The drawing under review shows one solid part. Ordinate dimensions are in mm from its lowest x, y, z. A direction names the side the tool comes from. Give positions to 0.01 mm unless a question says otherwise; leave off trailing zeros. Loops run counter-clockwise (first coordinate to the right, second up) from the corner with the lowest first, then second, coordinate; pieces in that order, holes last.
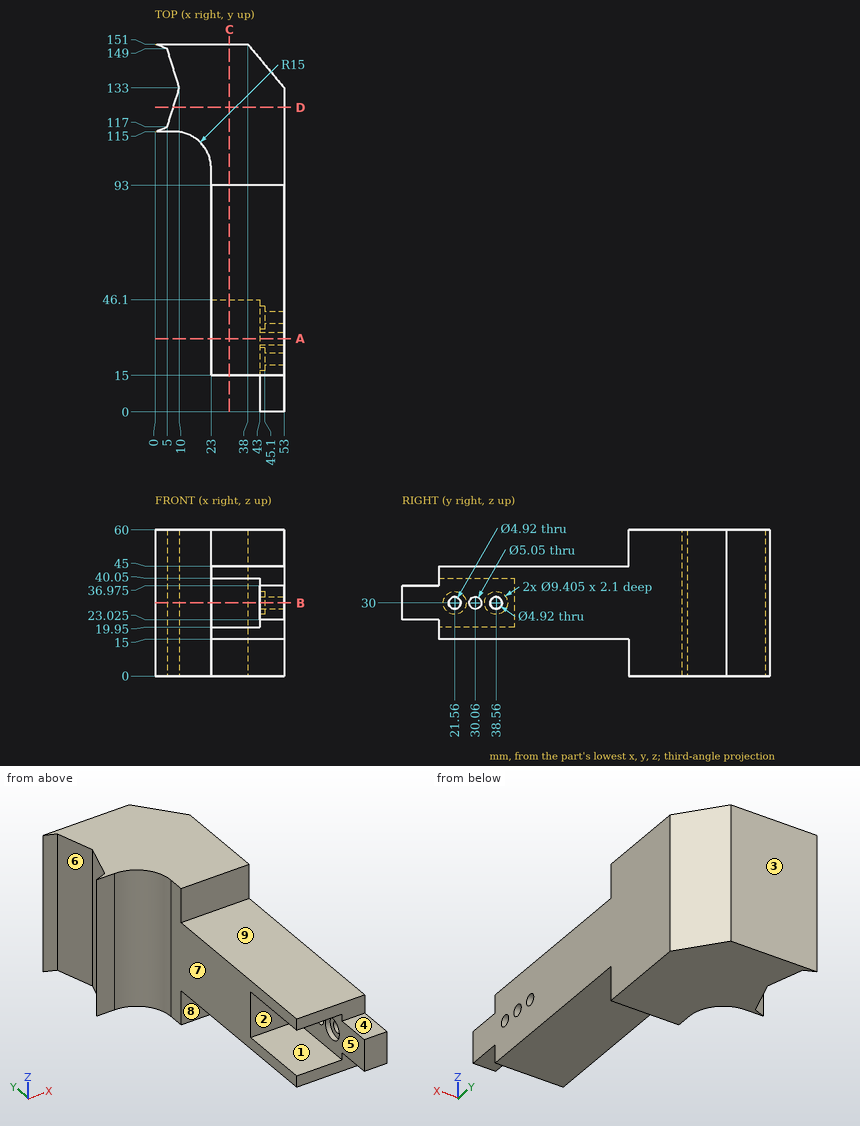
Item 1: Take a section at B-B on z = 30. State how many separate pieces and enclosed holes the cut face has, and give its area (3 significant figures).
Answer:
separate pieces: 4
enclosed holes: 0
area: 3,930 mm2
Item 2: Clearance check with flat-ended pins moving along their axes: pin 1 Ø16 at (x, z) = (33, 30) entering from -Y; pin 2 Ø10 at (y, z) = (16, 26) entering from -X; pin 3 Ø5 at (x, y) = (49.5, 10.5) entering from +Z (3 decimals). State where each tip first meets the part, or that it passes through.
Answer:
pin 1: stops at y = 46.1
pin 2: stops at x = 43
pin 3: stops at z = 36.975
Item 3: Take a section at C-C on x = 30.5. Give the boundary of the cut face in (y, z), and give its area (3 significant figures).
Answer:
outline: (15, 15) - (93, 15) - (93, 0) - (151, 0) - (151, 60) - (93, 60) - (93, 45) - (15, 45) - (15, 40.05) - (46.1, 40.05) - (46.1, 19.95) - (15, 19.95) - close
area: 5,190 mm2
Item 4: Tool access review of the marked faces 5, 6, 7, 8 and 9: name each direction out of +Z, -Z, +X, -X, +Y, -Y from which nothing blocks a thin tool from reaching the whole face with its end or side.
Answer:
face 5: -X, -Y
face 6: +Z, -Z, -X
face 7: +Z, -Z, -X, -Y
face 8: -Z, +X, -X, -Y
face 9: +Z, +X, -X, -Y
Item 5: Take a section at D-D on y = 125. Give the boundary of the cut face in (x, z).
Answer:
outline: (7.5, 0) - (53, 0) - (53, 60) - (7.5, 60) - close
Item 6: For L1, parallel to Y at x = 49.5, z = 30 (3 decimals); L2, parallel to Y at x = 47.25, z = 30 (3 decimals); L3, parallel to Z at x = 47.5, y = 38.56, list the stretches that pass through material, from the lowest coordinate up.
Answer:
L1: y = 0 to 19.1, 24.02 to 27.535, 32.585 to 36.1, 41.02 to 137.2
L2: y = 0 to 19.1, 24.02 to 27.535, 32.585 to 36.1, 41.02 to 139.9
L3: z = 15 to 27.54, 32.46 to 45
Item 7: Take a section at A-A on y = 30.06. Give the boundary of the cut face in (x, z) (3 decimals), and give its area (4 significant figures).
Answer:
outline: (23, 15) - (53, 15) - (53, 27.475) - (43, 27.475) - (43, 19.95) - (23, 19.95) - close; (23, 40.05) - (43, 40.05) - (43, 32.525) - (53, 32.525) - (53, 45) - (23, 45) - close
area: 447.5 mm2
Item 8: The part is to be moulded in two halves that separate along Z. For the marked faces 1, 2, 3 and 4, say which applies: released by +Z, released by -Z, zero draft, split by the parting line, or undercut.
Answer:
face 1: undercut
face 2: undercut
face 3: zero draft
face 4: released by +Z
